Read the model definition and answer for the solid it produces. Units are mm, in the model's axes. Face numbers are marked on the shaded views. Coordinates: 2 decimals unless noted, no trailing zeros. Write each loop counter-clockwise with the first axis right and the second up, starting at its lowest first coordinate (ties: lowest second). Pieces come first, ordered by that corner, then holes.
(1) The part is cut by section A-A, the plane z = 349.5. Determine the outline of the cut face in (x, y).
(2) The part is cut by section B-B, the plane x = 210. Determine the outline of the cut face in (y, z), and give its area (3 significant figures).
(3) Given pin 1 (5.5 mm diameter, centred on x = 210, y = 50, fed in from +Z); pin 2 (1.5 mm diameter, centred on x = 230, z = 346.5, fed in from +Y); pin 3 (4.5 mm diameter, centred on x = 230, y = 50, fed in from -Z), each flat-ended and moving along its own axis, determine where each tip first touches the part or whether it passes through.
(4) The part is cut by section C-C, the plane y = 50. Determine the outline of the cut face in (x, z) (3 decimals), and give its area (3 significant figures).
(5) Straight lines are drawn through the part: line 1 along X through (y, z) = (70, 344.25); line 2 along Y through (x, z) = (190, 346); line 3 along Y through (x, z) = (196.4, 348.25). For each, find the intervals that lie inside material, in ascending order.
(6) Determine the mould class of the marked faces 1, 2, 3 and 4 for opening direction Y: pulls with the +Y half, pulls with the -Y half, needs draft (parallel to the pull), parting line crosses it, or undercut.
(7) The part is cut by section D-D, the plane z = 341.25. Determine the outline of the cut face in (x, y).
```python
from build123d import *

# Parameters (mm, degrees)
SKETCH120_W     = 80
SKETCH120_H     = 50
SKETCH120_R     = 2.5
SKETCH120_R_2   = 5.5
PAD038_DEPTH    = 12
SKETCH121_R     = 2.5
POCKET077_DEPTH = 11
SKETCH122_R     = 8.05
POCKET078_DEPTH = 4.5
SKETCH123_R     = 4.6
SKETCH123_R_2   = 4.624594
SKETCH123_R_3   = 4.583454
SKETCH123_R_4   = 4.624604
POCKET079_DEPTH = 1.55


with BuildPart() as part:
    # Sketch120 → Pad038 (new body)
    with BuildSketch(Plane(origin=(260, 40, 352), x_dir=(-1, 0, 0), z_dir=(0, 0, -1))):
        with Locations((40, 25)):
            Rectangle(SKETCH120_W, SKETCH120_H)
        with Locations((10, 30)):
            Circle(SKETCH120_R, mode=Mode.SUBTRACT)
        with Locations((30, 10)):
            Circle(SKETCH120_R, mode=Mode.SUBTRACT)
        with Locations((16.4, 8.9)):
            Circle(SKETCH120_R, mode=Mode.SUBTRACT)
        with Locations((50, 10)):
            Circle(SKETCH120_R, mode=Mode.SUBTRACT)
        with Locations((63.6, 8.9)):
            Circle(SKETCH120_R, mode=Mode.SUBTRACT)
        with Locations((70, 30)):
            Circle(SKETCH120_R, mode=Mode.SUBTRACT)
        with Locations((40, 32.4)):
            Circle(SKETCH120_R_2, mode=Mode.SUBTRACT)
    extrude(amount=PAD038_DEPTH)

    # Sketch121 → Pocket077 (cut)
    with BuildSketch(Plane(origin=(260, 90, 352), x_dir=(1, 0, 0), z_dir=(0, 1, 0))):
        with Locations((-30.033846, 5.850095)):
            Circle(SKETCH121_R)
        with Locations((-50.003807, 5.788844)):
            Circle(SKETCH121_R)
    extrude(amount=-POCKET077_DEPTH, mode=Mode.SUBTRACT)

    # Sketch122 → Pocket078 (cut)
    with BuildSketch(Plane(origin=(260, 40, 340), x_dir=(-1, 0, 0), z_dir=(0, 0, -1))):
        with Locations((40, 32.4)):
            Circle(SKETCH122_R)
    extrude(amount=-POCKET078_DEPTH, mode=Mode.SUBTRACT)

    # Sketch123 → Pocket079 (cut)
    with BuildSketch(Plane(origin=(260, 40, 352), x_dir=(-1, 0, 0), z_dir=(0, 0, 1))):
        with Locations((10, -30)):
            Circle(SKETCH123_R)
        with Locations((70, -30)):
            Circle(SKETCH123_R_2)
        with Locations((30, -10)):
            Circle(SKETCH123_R_3)
        with Locations((50, -10)):
            Circle(SKETCH123_R_4)
    extrude(amount=-POCKET079_DEPTH, mode=Mode.SUBTRACT)


solid = part.part
```
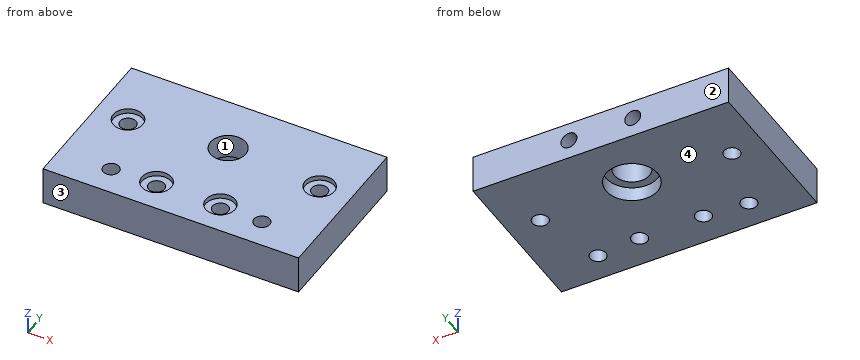
Computed:
1. outline: (180, 40) - (260, 40) - (260, 90) - (180, 90) - close; hole circle Ø5 at (190, 70); hole circle Ø5 at (196.4, 48.9); hole circle Ø5 at (210, 50); hole circle Ø11 at (220, 72.4); hole circle Ø5 at (230, 50); hole circle Ø5 at (243.6, 48.9); hole circle Ø5 at (250, 70)
2. outline: (40, 340) - (47.5, 340) - (47.5, 350.45) - (45.38, 350.45) - (45.38, 352) - (40, 352) - close; (52.5, 340) - (90, 340) - (90, 343.71) - (79, 343.71) - (79, 348.71) - (90, 348.71) - (90, 352) - (54.62, 352) - (54.62, 350.45) - (52.5, 350.45) - close
2. area: 478 mm2
3. pin 1: stops at z = 350.45
3. pin 2: stops at y = 79
3. pin 3: passes through
4. outline: (180, 340) - (194.155, 340) - (194.155, 352) - (180, 352) - close; (198.645, 340) - (207.5, 340) - (207.5, 350.45) - (205.375, 350.45) - (205.375, 352) - (198.645, 352) - close; (212.5, 340) - (227.5, 340) - (227.5, 350.45) - (225.417, 350.45) - (225.417, 352) - (214.625, 352) - (214.625, 350.45) - (212.5, 350.45) - close; (232.5, 340) - (241.355, 340) - (241.355, 352) - (234.583, 352) - (234.583, 350.45) - (232.5, 350.45) - close; (245.845, 340) - (260, 340) - (260, 352) - (245.845, 352) - close
4. area: 719 mm2
5. line 1: x = 180 to 187.5, 192.5 to 212.32, 227.68 to 247.5, 252.5 to 260
5. line 2: y = 40 to 67.5, 72.5 to 90
5. line 3: y = 40 to 46.4, 51.4 to 90
6. face 1: undercut
6. face 2: pulls with the +Y half
6. face 3: pulls with the -Y half
6. face 4: needs draft
7. outline: (180, 40) - (260, 40) - (260, 90) - (180, 90) - close; hole circle Ø5 at (190, 70); hole circle Ø5 at (196.4, 48.9); hole circle Ø5 at (210, 50); hole circle Ø16.1 at (220, 72.4); hole circle Ø5 at (230, 50); hole circle Ø5 at (243.6, 48.9); hole circle Ø5 at (250, 70)
